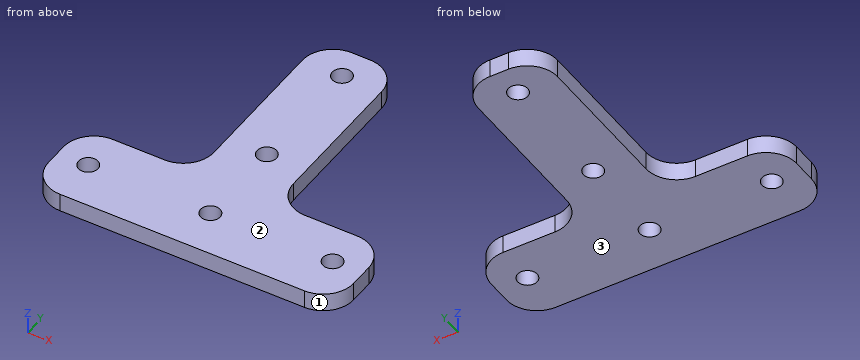
```python
from build123d import *

# Parameters (mm, degrees)
SKETCH_1_R      = 1.6
EXTRUDE_1_DEPTH = 3
FILLET_1_R      = 5


with BuildPart() as part:
    # 草图1 → 凸台-拉伸1 (new body)
    with BuildSketch(Plane.XY):
        Polygon((-6.5, 6.5), (-25, 6.5), (-25, -7.5), (25, -7.5), (25, 6.5), (6.5, 6.5), (6.5, 40), (-6.5, 40), align=None)
        with Locations((0, 35)):
            Circle(SKETCH_1_R, mode=Mode.SUBTRACT)
        with Locations((0, 15)):
            Circle(SKETCH_1_R, mode=Mode.SUBTRACT)
        Circle(SKETCH_1_R, mode=Mode.SUBTRACT)
        with Locations((20, 0)):
            Circle(SKETCH_1_R, mode=Mode.SUBTRACT)
        with Locations((-20, 0)):
            Circle(SKETCH_1_R, mode=Mode.SUBTRACT)
    extrude(amount=EXTRUDE_1_DEPTH)

    # 圆角1
    fillet_1_edges = [part.edges().sort_by_distance(p)[0] for p in [
        (-6.5, 40, 1.5),
        (6.5, 40, 1.5),
        (6.5, 6.5, 1.5),
        (25, 6.5, 1.5),
        (25, -7.5, 1.5),
        (-25, -7.5, 1.5),
        (-25, 6.5, 1.5),
        (-6.5, 6.5, 1.5),
    ]]
    fillet(fillet_1_edges, radius=FILLET_1_R)


solid = part.part
```
Build history of the part. All positions in model axes, mm. Face numbers are marked on the shaded views. Round coordinates to 2 decimals unless told otherwise and drop trailing zeros. Write each loop counter-clockwise with the first axis right and the second up, starting at its lowest first coordinate (ties: lowest second). Pieces come first, ordered by that corner, then holes. Notation, with made-up numbers: (4, -10) - (11, -10) arc R32 ccw to (11, 19) - close; hole circle Ø7 at (59.25, 63.25). An arc over 180 degrees is marked (long way). Answer as CSV lines item,"result".
Q1. Pull direction Z, two halves, no side cores. Call the marked faces 1, 2 and 3: +Z half, -Z half, draft (parallel to the pull), parting line (faces both ways), or undercut.
Report:
face 1,"draft"
face 2,"+Z half"
face 3,"-Z half"
Q2. Drop flat-ended pins along their axis: pin 1 (3 mm diameter, centred on x = -20, y = 0, fed in from +Z); pin 2 (12 mm diameter, centred on x = -7, y = 23, fed in from -Z). Give the stop position or say it passes through.
Report:
pin 1,"passes through"
pin 2,"stops at z = 0"
Q3. Cut at D-D (y = 0). Write the cut outline in (x, z), and give its area (3 significant figures).
Report:
outline,"(-25, 0) - (-21.6, 0) - (-21.6, 3) - (-25, 3) - close; (-18.4, 0) - (-1.6, 0) - (-1.6, 3) - (-18.4, 3) - close; (1.6, 0) - (18.4, 0) - (18.4, 3) - (1.6, 3) - close; (21.6, 0) - (25, 0) - (25, 3) - (21.6, 3) - close"
area,"121 mm^2"
Q4. Cut at B-B (z = 0.6). Write the cut outline in (x, y), and give its area (3 significant figures).
Report:
outline,"(-25, -2.5) arc R5 ccw to (-20, -7.5) - (20, -7.5) arc R5 ccw to (25, -2.5) - (25, 1.5) arc R5 ccw to (20, 6.5) - (11.5, 6.5) arc R5 cw to (6.5, 11.5) - (6.5, 35) arc R5 ccw to (1.5, 40) - (-1.5, 40) arc R5 ccw to (-6.5, 35) - (-6.5, 11.5) arc R5 cw to (-11.5, 6.5) - (-20, 6.5) arc R5 ccw to (-25, 1.5) - close; hole circle Ø3.2 at (-20, 0); hole circle Ø3.2 at (0, 0); hole circle Ø3.2 at (0, 15); hole circle Ø3.2 at (0, 35); hole circle Ø3.2 at (20, 0)"
area,"1,070 mm^2"
Q5. Drill centre lines: probe 1 along Y at (x, z) = (0, 1.2); probe 2 along Y at (x, z) = (1, 0.6); probe 3 along Y at (x, z) = (20, 2.1). Where is each one in solid material? Low to high. Write a range as [from, to].
Report:
probe 1,"y = [-7.5, -1.6], [1.6, 13.4], [16.6, 33.4], [36.6, 40]"
probe 2,"y = [-7.5, -1.25], [1.25, 13.75], [16.25, 33.75], [36.25, 40]"
probe 3,"y = [-7.5, -1.6], [1.6, 6.5]"
Q6. Cut at A-A (y = 15). Write the cut outline in (x, z), and give its area (3 significant figures).
Report:
outline,"(-6.5, 0) - (-1.6, 0) - (-1.6, 3) - (-6.5, 3) - close; (1.6, 0) - (6.5, 0) - (6.5, 3) - (1.6, 3) - close"
area,"29.4 mm^2"
Q7. Cut at C-C (x = 0). Write the cut outline in (y, z), and give its area (3 significant figures).
Report:
outline,"(-7.5, 0) - (-1.6, 0) - (-1.6, 3) - (-7.5, 3) - close; (1.6, 0) - (13.4, 0) - (13.4, 3) - (1.6, 3) - close; (16.6, 0) - (33.4, 0) - (33.4, 3) - (16.6, 3) - close; (36.6, 0) - (40, 0) - (40, 3) - (36.6, 3) - close"
area,"114 mm^2"
